Check sheet for the modelled part. Datum: model origin and axes. Units: mm. A direction names the side the tool comes from. Give positions to 0.01 mm unless a question says otherwise; leave off trailing zeros. Loops run counter-clockwise (first coordinate to the right, second up) from the corner with the lowest first, then second, coordinate; pieces in that order, holes last. Notation, with made-up numbers: M -17.75,51.5 L -9.75,51.5 A22 cw -9.75,77.5 Z; hole C -15,25 d3. An arc over 180 degrees is marked long. One line per question, with ' | ' between items. Start each with the question number.
Autodesk Fusion 360 part; units mm, degrees
sketch "Sketch1" plane through (0, 0, 0) normal (0, 0, 1) x (1, 0, 0)
  line L0 (0, 0) -> (75, 0)
  line L1 (75, 0) -> (75, 140)
  line L2 (75, 140) -> (0, 140)
  line L3 (0, 140) -> (0, 0)
  line L4 (0, 140) -> (-3, 140)
  line L5 (-3, 140) -> (-3, 0)
  line L6 (-3, 0) -> (0, 0)
  line L7 (0, 0) -> (0, 140)
  line L8 (75, 140) -> (78, 140)
  line L9 (78, 140) -> (78, 0)
  line L10 (78, 0) -> (75, 0)
  line L11 (75, 0) -> (75, 140)
  dimension "d1" = 140
  dimension "d2" = 75
  dimension "d3" = 3
  dimension "d4" = 3
extrude "Extrude1" add sketch "Sketch1" along normal blind 3 contours L0 L1 L2 L3 L7 L11
sketch "Sketch2" plane through (0, 0, 0) normal (0, 0, 1) x (1, 0, 0)
extrude "Extrude2" add sketch "Sketch1" along normal blind 40 contours L3 L4 L5 L6 L7 | L1 L8 L9 L10 L11
sketch "Sketch3" plane through (78, 0, 0) normal (1, 0, 0) x (0, 1, 0)
  line L0 (0, 0) -> (140, 0)
  line L1 (140, 0) -> (140, 40)
  line L2 (140, 40) -> (0, 40)
  line L3 (0, 40) -> (0, 0)
  line L4 (140, 0) -> (0, 0)
  line L5 (70, 40) -> (70, 0) construction
  line L6 (17.5, 40) -> (22.5, 40)
  line L7 (22.5, 40) -> (22.5, 37)
  line L8 (20.5, 35) -> (19.5, 35)
  line L9 (17.5, 37) -> (17.5, 40)
  arc A0 (17.5, 37) -> (19.5, 35) centre (19.5, 37) ccw
  arc A1 (20.5, 35) -> (22.5, 37) centre (20.5, 37) ccw
  line L10 (20, 40) -> (20, 35) construction
  line L11 (117.5, 40) -> (122.5, 40)
  line L12 (122.5, 40) -> (122.5, 37)
  line L13 (120.5, 35) -> (119.5, 35)
  line L14 (117.5, 37) -> (117.5, 40)
  arc A2 (117.5, 37) -> (119.5, 35) centre (119.5, 37) ccw
  arc A3 (120.5, 35) -> (122.5, 37) centre (120.5, 37) ccw
  line L15 (120, 35) -> (120, 40) construction
  point P0 (17.5, 35)
  point P1 (117.5, 35)
  dimension "d18" = 5
  dimension "d19" = 5
  dimension "d20" = 2
  dimension "d21" = 2
  dimension "d23" = 5
  dimension "d24" = 2
  dimension "d25" = 2
  dimension "d26" = 5
  dimension "d27" = 100
extrude "Extrude3" cut sketch "Sketch3" along normal mid plane 200 contours L2 L6 L7 L8 L9 A0 A1 | L2 L11 L12 L13 L14 A2 A3
Q1. Access from +Z, -Z, +X, -X, +Y, -Y to the whole of each face (thin tool, end or side, straight path). Record for faces 4 (the flat face through (76, 22.5, 39)), 5 (the flat face through (78, 71, 20)), 6 (the flat face through (37, 71, 3)).
Q2. Cross-section at C-C (x = 36). Record the cut outline in (y, z), and give its area (3 significant figures).
Q3. Material ranges on probe 1 along X at (y, z) = (28, 14); probe 2 along Z at (x, y) = (18, 96), recorded low to high. Write a range as from..to.
Q4. Cross-section at B-B (y = 110). Record the cut outline in (x, z), and give its area (3 significant figures).
Q5. Draft check along Y on faces 1 (the flat face through (76, 71, 40)), 2 (the flat face through (41, 140, 2)), 3 (the flat face through (-2, 122.5, 39)). Enter one of: released by +Y, released by -Y, zero draft, split by the parting line, or undercut.
Q6. Depth check by flat-ended pin: P1, Ø2, axis at x = 57.5, y = 47.5, coming from the -Z side; P2, Ø1.1, axis at x = 77, y = 20, coming from the +Z side. Enter the tip coordinate at first touch or a pass-through.
Q7. Cross-section at A-A (z = 31). Record the cut outline in (x, y).
Solved:
1) face 4: +Z, +X, -X | face 5: +Z, -Z, +X, +Y, -Y | face 6: +Z, +Y, -Y
2) outline: M 0,0 L 140,0 L 140,3 L 0,3 Z | area: 420 mm²
3) probe 1: x = -3..0, 75..78 | probe 2: z = 0..3
4) outline: M -3,0 L 78,0 L 78,40 L 75,40 L 75,3 L 0,3 L 0,40 L -3,40 Z | area: 465 mm²
5) face 1: zero draft | face 2: released by +Y | face 3: undercut
6) P1: stops at z = 0 | P2: stops at z = 35
7) outline: M -3,0 L 0,0 L 0,140 L -3,140 Z; M 75,0 L 78,0 L 78,140 L 75,140 Z
